Check sheet for the modelled part. Datum: model origin and axes. Units: mm. Face numbers are marked on the shaded views. A direction names the side the tool comes from. Give positions to 0.01 mm unless a question says otherwise; leave off trailing zeros. Order: outer loops, then holes, each group sorted by start corner. A loop starts at its lowest first (then second) coordinate and runs counter-clockwise, first axis right, second up. Notation, with made-up numbers: (-4, 2) -> (48, 2) arc R18 ccw to (48, 28) -> close; hole circle Ø5 at (-21.75, 0.5). An arc over 180 degrees is marked (long way). One line per question, with ' | ' between items.
```python
from build123d import *

# Parameters (mm, degrees)
BOSS_EXTRUDE1_DEPTH = 15
CUT_EXTRUDE1_DEPTH  = 21.4450483
SKETCH3_W           = 7
SKETCH3_H           = 7.5
CUT_EXTRUDE2_DEPTH  = 21.4450483


with BuildPart() as part:
    # Sketch1 → Boss-Extrude1 (new body)
    with BuildSketch(Plane(origin=(0, 0, 0), x_dir=(1, 0, 0), z_dir=(0, 1, 0))):
        with BuildLine():
            ThreePointArc((0, 2.5), (1.767766953, 1.767766953), (2.5, 0))
            Line((2.5, 0), (3.5, 0))
            ThreePointArc((3.5, 0), (2.474873734, 2.474873734), (0, 3.5))
            Line((0, 3.5), (0, 2.5))
        make_face()
        with BuildLine():
            Line((-3.5, 0), (-2.5, 0))
            ThreePointArc((-2.5, 0), (-1.767766953, 1.767766953), (0, 2.5))
            Line((0, 2.5), (0, 3.5))
            ThreePointArc((0, 3.5), (-2.474873734, 2.474873734), (-3.5, 0))
        make_face()
        with BuildLine():
            Line((0, -5.5), (0, -2.5))
            ThreePointArc((0, -2.5), (-1.767766953, -1.767766953), (-2.5, 0))
            Line((-2.5, 0), (-3.5, 0))
            Line((-3.5, 0), (-3.5, -3.5))
            Line((-3.5, -3.5), (-12, -3.5))
            Line((-12, -3.5), (-12, -5.5))
            Line((-12, -5.5), (0, -5.5))
        make_face()
        with BuildLine():
            ThreePointArc((2.5, 0), (1.767766953, -1.767766953), (0, -2.5))
            Line((0, -2.5), (0, -5.5))
            Line((0, -5.5), (12, -5.5))
            Line((12, -5.5), (12, -3.5))
            Line((12, -3.5), (3.5, -3.5))
            Line((3.5, -3.5), (3.5, 0))
            Line((3.5, 0), (2.5, 0))
        make_face()
    extrude(amount=BOSS_EXTRUDE1_DEPTH)

    # Sketch2 → Cut-Extrude1 (cut, through all)
    with BuildSketch(Plane(origin=(0, 0, 3.5), x_dir=(-1, 0, 0), z_dir=(0, 0, -1))):
        with BuildLine():
            ThreePointArc((-6.25, 7.5), (-6.689339828, 8.560660172), (-7.75, 9))
            Line((-7.75, 9), (-7.75, 6))
            ThreePointArc((-7.75, 6), (-6.689339828, 6.439339828), (-6.25, 7.5))
        make_face()
        with BuildLine():
            Line((-7.75, 6), (-7.75, 9))
            ThreePointArc((-7.75, 9), (-9.25, 7.5), (-7.75, 6))
        make_face()
        with BuildLine():
            ThreePointArc((9.25, 7.5), (8.810660172, 8.560660172), (7.75, 9))
            Line((7.75, 9), (7.75, 6))
            ThreePointArc((7.75, 6), (8.810660172, 6.439339828), (9.25, 7.5))
        make_face()
        with BuildLine():
            Line((7.75, 6), (7.75, 9))
            ThreePointArc((7.75, 9), (6.25, 7.5), (7.75, 6))
        make_face()
    extrude(amount=-CUT_EXTRUDE1_DEPTH, mode=Mode.SUBTRACT)

    # Sketch3 → Cut-Extrude2 (cut, through all)
    with BuildSketch(Plane(origin=(0, 0, 3.5), x_dir=(-1, 0, 0), z_dir=(0, 0, -1))):
        with Locations((0, 3.75)):
            Rectangle(SKETCH3_W, SKETCH3_H)
    extrude(amount=CUT_EXTRUDE2_DEPTH, mode=Mode.SUBTRACT)


solid = part.part
```
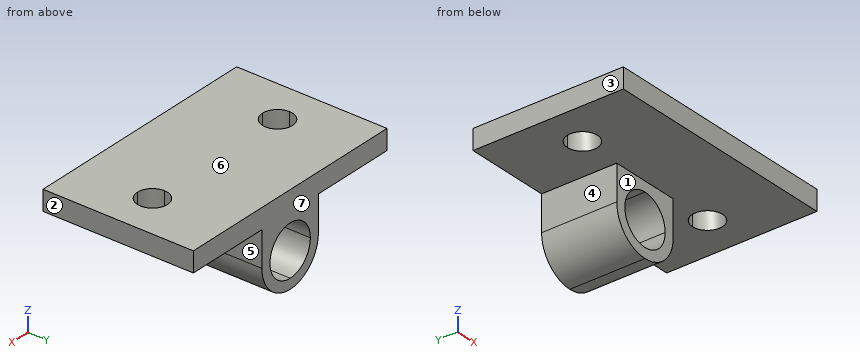
Q1. Access from +Z, -Z, +X, -X, +Y, -Y to the whole of each face (thin tool, end or side, straight path). Record for the marked faces 1, 2, 3, 4 and 5.
Result sheet:
face 1: -Z, +X, -X, -Y | face 2: +Z, -Z, +X, +Y, -Y | face 3: +Z, -Z, -X, +Y, -Y | face 4: -Z, -X, +Y, -Y | face 5: -Z, +X, +Y, -Y
Q2. Section check A-A (z = 1.5). Enter the section's corners in (x, y).
Result sheet:
outline: (-3.5, 7.5) -> (-2, 7.5) -> (-2, 15) -> (-3.5, 15) -> close; (2, 7.5) -> (3.5, 7.5) -> (3.5, 15) -> (2, 15) -> close
Q3. Section check C-C (y = 11). Enter the section's corners in (x, z).
Result sheet:
outline: (-12, 3.5) -> (-3.5, 3.5) -> (-3.5, 0) arc R3.5 ccw to (3.5, 0) -> (3.5, 3.5) -> (12, 3.5) -> (12, 5.5) -> (-12, 5.5) -> close; hole circle Ø5 at (0, 0)
Q4. Thickness scan on line 1 (X direction, y = 8, z = 4.5); line 2 (Z direction, x = -1, y = 6); line 3 (Y direction, x = -9, z = 5.25). Record the ranges inside material, lowest first.
Result sheet:
line 1: x = -12 to -9.16, -6.34 to 6.34, 9.16 to 12 | line 2: z = 3.5 to 5.5 | line 3: y = 0 to 6.67, 8.33 to 15
Q5. Mould release check, pull along Z, two halves, no side actions. Record for the marked faces 6 and 7: pulls with the +Z half, pulls with the -Z half, needs draft (parallel to the pull), parting line crosses it, or undercut.
Result sheet:
face 6: pulls with the +Z half | face 7: needs draft
Q6. Section check B-B (y = 8). Enter the section's corners in (x, z).
Result sheet:
outline: (-12, 3.5) -> (-9.16, 3.5) -> (-9.16, 5.5) -> (-12, 5.5) -> close; (-6.34, 3.5) -> (-3.5, 3.5) -> (-3.5, 0) arc R3.5 ccw to (3.5, 0) -> (3.5, 3.5) -> (6.34, 3.5) -> (6.34, 5.5) -> (-6.34, 5.5) -> close; (9.16, 3.5) -> (12, 3.5) -> (12, 5.5) -> (9.16, 5.5) -> close; hole circle Ø5 at (0, 0)
Q7. Section check D-D (z = 3.75). Enter the section's corners in (x, y).
Result sheet:
outline: (-12, 0) -> (12, 0) -> (12, 15) -> (-12, 15) -> close; hole circle Ø3 at (-7.75, 7.5); hole circle Ø3 at (7.75, 7.5)
Q8. Depth check by flat-ended pin: pin 1 Ø1.5 at (x, z) = (-9, 2.5) entering from +Y; pin 2 Ø4 at (y, z) = (12, 1) entering from -X; pin 3 Ø3 at (x, y) = (-0.5, 1.5) entering from -Z; pin 4 Ø7.5 at (x, y) = (3.5, 5) entering from -Z. Enter the tip coordinate at first touch or a pass-through.
Result sheet:
pin 1: passes through | pin 2: stops at x = -3.5 | pin 3: stops at z = 3.5 | pin 4: stops at z = -3.43
